Verification items for this drawing (mm, ordinates from the low corner). A direction names the side the tool comes from. Coordinates: 2 decimals unless noted, no trailing zeros. Loops run counter-clockwise (first coordinate to the right, second up) from the corner with the lowest first, then second, coordinate; pieces in that order, holes last. Notation, with made-up numbers: M 27.25,1 L 51.25,1 A24 ccw 51.25,36 Z; hole C -2.75,-24 d5. An arc over 180 degrees is marked long. Return JSON: item names as keys, results as strings.
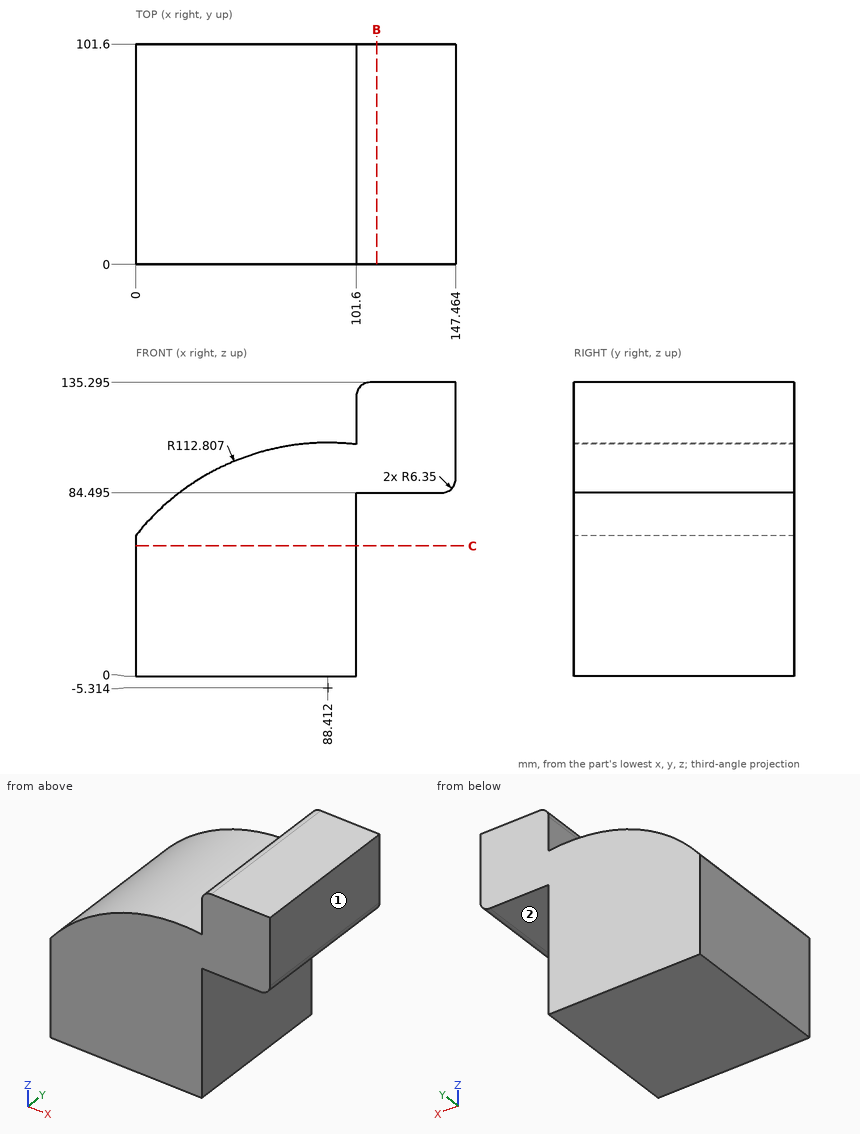
1) Section check B-B on x = 111. Record the cut outline in (y, z) (1 decimal), then the cut area to 3 significant figures.
Answers:
{"outline": "M 0,84.5 L 101.6,84.5 L 101.6,135.3 L 0,135.3 Z", "area": "5,160 mm²"}
2) Scan lines: line 1 along Z through (x, y) = (109, 40) (1 decimal); line 2 along X through (y, z) = (47, 54); line 3 along X through (y, z) = (70, 124.5). Record each from-to range of solid material in increasing order. Write a range as [from, to].
Answers:
{"line 1": "[84.5, 135.3]", "line 2": "[0, 101.6]", "line 3": "[101.6, 147.46]"}
3) Set-up check for the marked faces 1 and 2: record each of +Z, -Z, +X, -X, +Y, -Y from which the full face is reachable in a straight line by a thin tool's end or side.
Answers:
{"face 1": "+Z, -Z, +X, +Y, -Y", "face 2": "-Z, +X, +Y, -Y"}
4) Section check C-C on z = 60. Record the cut outline in (x, y).
Answers:
{"outline": "M 0,0 L 101.6,0 L 101.6,101.6 L 0,101.6 Z"}
5) Go/stop test with flat-tipped pins: pin 1 Ø3 at (x, y) = (43, 48) entering from +Z (1 decimal); pin 2 Ø1 at (y, z) = (31, 66.5) entering from +X; pin 3 Ø1.5 at (x, y) = (59, 71.5) entering from +Z. Record where each tip stops, or that it passes through.
Answers:
{"pin 1": "z = 98.6", "pin 2": "x = 101.6", "pin 3": "z = 103.79"}
